Read the model definition and answer for the solid it produces. Units are mm, in the model's axes. A direction names the side the tool comes from. Coordinates: 2 decimals unless noted, no trailing zeros. Write each loop counter-clockwise with the first axis right and the second up, starting at its lowest first coordinate (ties: lowest second). Pieces come first, ordered by that corner, then holes.
Item 1: A tool of negligible diameter and unlimited length cuts with its end or side. For faces 1 (the face through (10, 0, 0)), 2 (the face through (13, 44, -12.5)), 3 (the face through (-9.81, -52.6, 0.18)), 4 (the face through (-52.6, 9.81, 0.18)), 5 (the face through (-20.41, 49.27, 0.18)), from which of +Z, -Z, +X, -X, +Y, -Y can it reach the whole face along a straight path? Write none if from no direction.
Item 2: Determine the mould class of faces 6 (the face through (14, 0, -25)), 7 (the face through (54.538, -21.355, 0.175)), 8 (the face through (-7.21, -32.49, 24.22)) for opening direction X: released by +X, released by -X, zero draft, split by the parting line, or undercut.
Item 3: Straight lines are drawn through the part: probe 1 along Y at (x, z) = (-2, 10); probe 2 along Z at (x, y) = (37.5, 42); probe 3 along X at (y, z) = (-18.5, -14). For each, find the intervals that lie inside material, in ascending order.
Item 4: Each of these flat-tipped pins is pushed along its axis until it touches: P1, Ø7.5, axis at x = 52, z = 5, coming from the -Y side; P2, Ø12, axis at y = -36, z = -1.5, coming from the -X side; P3, Ø3.5, axis at y = 54, z = 4.5, coming from the +X side; P4, Ø8, axis at x = -0.5, z = -0.5, coming from the -Y side. Where does it stop, or does it pass through?
Item 5: Section A-A (z = 17) is taken. Give the vertices of the cut face in (x, y), then the cut area to 3 significant figures.
from build123d import *

# Parameters (mm, degrees)
F0_R       = 45
F0_W       = 20
F0_H       = 50
F1_DEPTH   = 12.5
F2_DEPTH   = 25
F3_SIZE2   = 12.49999
F3_SIZE    = 12.49999
F4_SIZE    = 12.49999
F5_R       = 2
F6_SIZE2   = 20
F6_SIZE    = 3
F6_2_SIZE2 = 20
F6_2_SIZE  = 3
F7_SIZE2   = 3
F7_SIZE    = 20


# Not quite as in the source:
# - a fillet or chamfer is up to 0.001 mm smaller than in the source, because OpenCascade refuses the exact size


with BuildPart() as f1:
    # F0 (on Top) → F1 (new body, symmetric)
    with BuildSketch(Plane.XY):
        Polygon((46.1939766256, -19.1341716183), (50, 0), (46.1939766256, 19.1341716183), (35.3553390593, 35.3553390593), (19.1341716183, 46.1939766256), (0, 50), (-19.1341716183, 46.1939766256), (-35.3553390593, 35.3553390593), (-46.1939766256, 19.1341716183), (-50, 0), (-46.1939766256, -19.1341716183), (-35.3553390593, -35.3553390593), (-19.1341716183, -46.1939766256), (0, -50), (19.1341716183, -46.1939766256), (35.3553390593, -35.3553390593), align=None)
        Circle(F0_R, mode=Mode.SUBTRACT)
        Circle(F0_R)
        Rectangle(F0_W, F0_H, mode=Mode.SUBTRACT)
        Polygon((-19.1341716183, 46.1939766256), (0, 50), (0, 60.7945092961), align=None)
        Polygon((-35.3553390593, 35.3553390593), (-19.1341716183, 46.1939766256), (-23.2650514864, 56.1668028277), align=None)
        Polygon((-46.1939766256, 19.1341716183), (-35.3553390593, 35.3553390593), (-42.9882097822, 42.9882097822), align=None)
        Polygon((-50, 0), (-46.1939766256, 19.1341716183), (-56.1668028277, 23.2650514864), align=None)
        Polygon((-60.7945092961, 0), (-46.1939766256, -19.1341716183), (-50, 0), align=None)
        Polygon((-56.1668028277, -23.2650514864), (-35.3553390593, -35.3553390593), (-46.1939766256, -19.1341716183), align=None)
        Polygon((-42.9882097822, -42.9882097822), (-19.1341716183, -46.1939766256), (-35.3553390593, -35.3553390593), align=None)
        Polygon((-23.2650514864, -56.1668028277), (0, -50), (-19.1341716183, -46.1939766256), align=None)
        Polygon((0, -60.7945092961), (19.1341716183, -46.1939766256), (0, -50), align=None)
        Polygon((23.2650514864, -56.1668028277), (35.3553390593, -35.3553390593), (19.1341716183, -46.1939766256), align=None)
        Polygon((42.9882097822, -42.9882097822), (46.1939766256, -19.1341716183), (35.3553390593, -35.3553390593), align=None)
        Polygon((56.1668028277, -23.2650514864), (50, 0), (46.1939766256, -19.1341716183), align=None)
        Polygon((46.1939766256, 19.1341716183), (50, 0), (60.7945092961, 0), align=None)
        Polygon((35.3553390593, 35.3553390593), (46.1939766256, 19.1341716183), (56.1668028277, 23.2650514864), align=None)
        Polygon((19.1341716183, 46.1939766256), (35.3553390593, 35.3553390593), (42.9882097822, 42.9882097822), align=None)
        Polygon((0, 50), (19.1341716183, 46.1939766256), (23.2650514864, 56.1668028277), align=None)
    extrude(amount=F1_DEPTH, both=True)

    # F0 (on Top) → F2 (join, symmetric)
    with BuildSketch(Plane.XY):
        Circle(F0_R)
        Rectangle(F0_W, F0_H, mode=Mode.SUBTRACT)
    extrude(amount=F2_DEPTH, both=True)

    # F3 (size 12.5 and 12.5 in the source; OpenCascade refuses exactly that, so slightly less here)
    f3_edges = [f1.edges().sort_by_distance(p)[0] for p in [
        (-45, 0, 25),
    ]]
    chamfer(f3_edges, length=F3_SIZE, length2=F3_SIZE2)

    # F4 (size 12.5 in the source; OpenCascade refuses exactly that, so slightly less here)
    f4_edges = [f1.edges().sort_by_distance(p)[0] for p in [
        (-45, 0, -25),
    ]]
    chamfer(f4_edges, length=F4_SIZE)

    # F5
    f5_edges = [f1.edges().sort_by_distance(p)[0] for p in [
        (23.265051, 56.166803, 0),
        (0, 60.794509, 0),
        (-23.265051, 56.166803, 0),
        (-42.98821, 42.98821, 0),
        (-56.166803, 23.265051, 0),
        (-60.794509, 0, 0),
        (-56.166803, -23.265051, 0),
        (-42.98821, -42.98821, 0),
        (-23.265051, -56.166803, 0),
        (0, -60.794509, 0),
        (23.265051, -56.166803, 0),
        (42.98821, 42.98821, 0),
        (56.166803, 23.265051, 0),
        (60.794509, 0, 0),
        (56.166803, -23.265051, 0),
        (42.98821, -42.98821, 0),
    ]]
    fillet(f5_edges, radius=F5_R)

    # F6
    f6_edges = [f1.edges().sort_by_distance(p)[0] for p in [
        (0, 25, -25),
        (-10, 0, -25),
        (10, 0, -25),
        (0, -25, -25),
    ]]
    f6_side = f1.faces().sort_by_distance((-31.580771, 0, -25))[0]
    chamfer(f6_edges, length=F6_SIZE, length2=F6_SIZE2, reference=f6_side)

    # F6#2
    f6_2_edges = [f1.edges().sort_by_distance(p)[0] for p in [
        (-10, 0, 25),
        (0, -25, 25),
        (0, 25, 25),
    ]]
    f6_2_side = f1.faces().sort_by_distance((-31.580771, 0, 25))[0]
    chamfer(f6_2_edges, length=F6_2_SIZE, length2=F6_2_SIZE2, reference=f6_2_side)

    # F7
    f7_edges = [f1.edges().sort_by_distance(p)[0] for p in [
        (10, 0, 25),
    ]]
    f7_side = f1.faces().sort_by_distance((10, 0, 10.320513))[0]
    chamfer(f7_edges, length=F7_SIZE, length2=F7_SIZE2, reference=f7_side)


solid = f1.part
Established:
1. face 1: +Z, -Z
1. face 2: -Z
1. face 3: +Z, -Z, -Y
1. face 4: +Z, -Z, -X
1. face 5: +Z, -Z, +Y
2. face 6: zero draft
2. face 7: undercut
2. face 8: split by the parting line
3. probe 1: y = -50.53 to -25.75, 25.75 to 58.75
3. probe 2: z = -12.5 to 12.5
3. probe 3: x = -39.37 to -11.35, 11.35 to 39.37
4. P1: stops at y = -21.87
4. P2: stops at x = -44.57
4. P3: stops at x = 21.87
4. P4: stops at y = -58.75
5. outline: circle Ø81 at (0, 0); hole (-11.8, -26.8) - (11.8, -26.8) - (11.8, 26.8) - (-11.8, 26.8) - close
5. area: 3,890 mm2
